Work out the finished part from the listing and answer in its coordinate system (mm). A direction names the side the tool comes from. Round coordinates to 2 decimals unless told otherwise and drop trailing zeros. Write each loop counter-clockwise with the first axis right and the second up, starting at its lowest first coordinate (ties: lowest second). Pieces come first, ordered by that corner, then holes. Notation, with made-up numbers: M 62,66 L 101,66 A12 ccw 101,73 Z; hole C 33,57.25 d11. An arc over 180 degrees is marked long. One line per item, written item: value. Start each with the question number.
Q1. Find section C-C (z = 1.3). Write down the section's boundary in (x, y) (3 decimals).
Q2. Find section D-D (y = 38.5). Write down the section's boundary in (x, z) (3 decimals), and give its area (3 significant figures).
Q3. A tool of negligible diameter and unlimited length cuts with its end or side. For faces 1 (the flat face through (20, 20, 2)), 2 (the flat face through (105, 20, 2)), 3 (the flat face through (62, 0, 2)), from which of +Z, -Z, +X, -X, +Y, -Y can it reach the whole face along a straight path? Write none if from no direction.
Q4. Given pin 1 Ø4.5 at (x, y) = (10, 40) entering from +Z; pin 2 Ø1 at (x, z) = (116, 1.5) entering from -Y; pin 3 Ø1 at (x, y) = (74, 34) entering from -Z, each flat-ended and moving along its own axis, determine where each tip first touches the part or whether it passes through.
Q5. Consider probe 1 along Y at (x, z) = (115, 1.2); probe 2 along X at (y, z) = (42, 1.05); probe 3 along X at (y, z) = (24.5, 2.8). Determine where each line is inside the solid, lowest interval first.
Q6. Find section B-B (y = 20). Write down the section's boundary in (x, z) (3 decimals), and give its area (3 significant figures).
Q7. Find section A-A (x = 115). Write down the section's boundary in (y, z) (3 decimals).
Q8. The mould has two halves that part along Y. Classify faces 4 (the flat face through (115, 30, 2)), 5 (the cylindrical face through (75.686, 14.533, 1.61)), 6 (the flat face through (62, 36, 3.175)), 7 (the cylindrical face through (10.358, 42.727, 1.565)): released by +Y, released by -Y, zero draft, split by the parting line, or undercut.
from build123d import *

# Parameters (mm, degrees)
SKETCH1_W           = 125
SKETCH1_H           = 50
BOSS_EXTRUDE1_DEPTH = 3.175
SKETCH2_R           = 14.275
CUT_EXTRUDE1_DEPTH  = 4.175
SKETCH6_R           = 2.75
SKETCH6_W           = 20
SKETCH6_H           = 30
CUT_EXTRUDE6_DEPTH  = 4.175
FILLET1_R           = 10


with BuildPart() as part:
    # Sketch1 → Boss-Extrude1 (new body)
    with BuildSketch(Plane.XY):
        with Locations((62.5, 25)):
            Rectangle(SKETCH1_W, SKETCH1_H)
    extrude(amount=BOSS_EXTRUDE1_DEPTH)

    # Sketch2 → Cut-Extrude1 (cut, through all)
    with BuildSketch(Plane.XY.offset(3.175)):
        with Locations((62.5, 20)):
            Circle(SKETCH2_R)
    extrude(amount=-CUT_EXTRUDE1_DEPTH, mode=Mode.SUBTRACT)

    # Sketch6 → Cut-Extrude6 (cut, through all)
    with BuildSketch(Plane(origin=(0, 0, 0), x_dir=(-1, 0, 0), z_dir=(0, 0, -1))):
        with Locations((-115, 40)):
            Circle(SKETCH6_R)
        with Locations((-10, 40)):
            Circle(SKETCH6_R)
        with Locations((-115, 15)):
            Rectangle(SKETCH6_W, SKETCH6_H)
        with Locations((-10, 15)):
            Rectangle(SKETCH6_W, SKETCH6_H)
    extrude(amount=-CUT_EXTRUDE6_DEPTH, mode=Mode.SUBTRACT)

    # Fillet1
    fillet1_edges = [part.edges().sort_by_distance(p)[0] for p in [
        (105, 0, 1.5875),
        (20, 0, 1.5875),
    ]]
    fillet(fillet1_edges, radius=FILLET1_R)


solid = part.part
The answers:
1. outline: M 0,30 L 20,30 L 20,10 A10 ccw 30,0 L 95,0 A10 ccw 105,10 L 105,30 L 125,30 L 125,50 L 0,50 Z; hole C 10,40 d5.5; hole C 62.5,20 d28.55; hole C 115,40 d5.5
2. outline: M 0,0 L 7.695,0 L 7.695,3.175 L 0,3.175 Z; M 12.305,0 L 112.695,0 L 112.695,3.175 L 12.305,3.175 Z; M 117.305,0 L 125,0 L 125,3.175 L 117.305,3.175 Z
2. area: 368 mm2
3. face 1: +Z, -Z, -X, -Y
3. face 2: +Z, -Z, +X, -Y
3. face 3: +Z, -Z, +X, -X, -Y
4. pin 1: through
4. pin 2: y = 30
4. pin 3: z = 0
5. probe 1: 30 to 37.25, 42.75 to 50
5. probe 2: 0 to 8.11, 11.89 to 113.11, 116.89 to 125
5. probe 3: 20 to 48.95, 76.05 to 105
6. outline: M 20,0 L 48.225,0 L 48.225,3.175 L 20,3.175 Z; M 76.775,0 L 105,0 L 105,3.175 L 76.775,3.175 Z
6. area: 179 mm2
7. outline: M 30,0 L 37.25,0 L 37.25,3.175 L 30,3.175 Z; M 42.75,0 L 50,0 L 50,3.175 L 42.75,3.175 Z
8. face 4: released by -Y
8. face 5: undercut
8. face 6: zero draft
8. face 7: undercut
